```python
from build123d import *

# Parameters (mm, degrees)
SKETCH1_W           = 40
SKETCH1_H           = 40
SKETCH1_W_2         = 30
SKETCH1_H_2         = 30
BOSS_EXTRUDE1_DEPTH = 450
SKETCH2_R           = 2.5
CUT_EXTRUDE1_DEPTH  = 450
CUT_EXTRUDE2_DEPTH  = 76
LPATTERN1_COUNT     = 5
LPATTERN1_PITCH     = 30


with BuildPart() as part:
    # Sketch1 → Boss-Extrude1 (new body)
    with BuildSketch(Plane.XY):
        Rectangle(SKETCH1_W, SKETCH1_H)
        Rectangle(SKETCH1_W_2, SKETCH1_H_2, mode=Mode.SUBTRACT)
    extrude(amount=BOSS_EXTRUDE1_DEPTH)

    # Sketch2 → Cut-Extrude1 (cut)
    with BuildSketch(Plane(origin=(20, 0, 0), x_dir=(0, 0, -1), z_dir=(1, 0, 0))):
        with Locations((-430, 0)):
            Circle(SKETCH2_R)
    cut_extrude1 = extrude(amount=-CUT_EXTRUDE1_DEPTH, mode=Mode.SUBTRACT)

    # Sketch3 → Cut-Extrude2 (cut)
    with BuildSketch(Plane(origin=(20, 0, 0), x_dir=(0, 0, -1), z_dir=(1, 0, 0))):
        with BuildLine():
            ThreePointArc((-450, 2.8e-07), (-444.142135525, 14.142135723), (-430, 20))
            Line((-430, 20), (-450, 20))
            Line((-450, 20), (-450, 2.8e-07))
        make_face()
        with BuildLine():
            ThreePointArc((-430, -20), (-444.142135723, -14.142135525), (-450, 2.8e-07))
            Line((-450, 2.8e-07), (-450, -20))
            Line((-450, -20), (-430, -20))
        make_face()
    extrude(amount=-CUT_EXTRUDE2_DEPTH, mode=Mode.SUBTRACT)

    # LPattern1: Cut-Extrude1 ×5
    with Locations(*[(0, 0, -i * LPATTERN1_PITCH) for i in range(1, LPATTERN1_COUNT)]):
        add(cut_extrude1, mode=Mode.SUBTRACT)


solid = part.part
```
For this review, take the finished solid that the model builds, in its own axes (mm). A direction names the side the tool comes from. Coordinates: 2 decimals unless noted, no trailing zeros. Loops run counter-clockwise (first coordinate to the right, second up) from the corner with the lowest first, then second, coordinate; pieces in that order, holes last. Notation, with made-up numbers: (61, 31.25) -> (95, 31.25) arc R11 cw to (95, 50.25) -> close; hole circle Ø7 at (62.25, -11). An arc over 180 degrees is marked (long way). Return JSON: item names as keys, results as strings. Group by question number.
(1) Tool access review of faces 5 (the flat face through (0, 15, 219)), 6 (the flat face through (-18, 0, 0)): name each direction out of +Z, -Z, +X, -X, +Y, -Y from which nothing blocks a thin tool from reaching the whole face with its end or side.
(2) Consider section C-C, the plane y = -8. Give the boundary of the cut face in (x, z), plus the area to 3 significant figures.
(3) Consider section B-B, the plane z = 134.5. Give the boundary of the cut face in (x, y).
(4) Consider section A-A, the plane x = -9. Give the boundary of the cut face in (y, z), plus the area to 3 significant figures.
(5) Mouldability with a two-part tool opening along Y and no side actions: class faces 1 (the flat face through (-15, 0, 222)), 2 (the flat face through (-20, 0, 222)), 3 (the flat face through (0, -15, 219)), 4 (the flat face through (0, 20, 212)) as pulls with the +Y half, pulls with the -Y half, needs draft (parallel to the pull), parting line crosses it, or undercut.
(6) To check wall thickness, follow L1, parallel to Y at x = -16, z = 430; L2, parallel to X at y = -2.5, z = 277.5. State the ranges of each line that lie inside material, in increasing order.
Results below:
{
 "1": {"face 5": "+Z, -Z", "face 6": "-Z, +X, -X, +Y, -Y"},
 "2": {"outline": "(-20, 0) -> (-15, 0) -> (-15, 448.33) -> (-20, 448.33) -> close; (15, 0) -> (20, 0) -> (20, 448.33) -> (15, 448.33) -> close", "area": "4,480 mm2"},
 "3": {"outline": "(-20, -20) -> (20, -20) -> (20, 20) -> (-20, 20) -> close; hole (-15, -15) -> (15, -15) -> (15, 15) -> (-15, 15) -> close"},
 "4": {"outline": "(-20, 0) -> (-15, 0) -> (-15, 443.23) arc R20 ccw to (-20, 430) -> close; (15, 0) -> (20, 0) -> (20, 430) arc R20 ccw to (15, 443.23) -> close", "area": "4,390 mm2"},
 "5": {"face 1": "undercut", "face 2": "needs draft", "face 3": "undercut", "face 4": "pulls with the +Y half"},
 "6": {"L1": "y = -20 to -2.5, 2.5 to 20", "L2": "x = -20 to -15, 15 to 20"}
}
